Design review of the part shown in the three views and the two pictorial views. Dimensions are in mm from the part's minimum x, y and z. A direction names the side the tool comes from. Coordinates: 2 decimals unless noted, no trailing zeros. Order: outer loops, then holes, each group sorted by start corner. A loop starts at its lowest first (then second) coordinate and runs counter-clockwise, first axis right, second up. Notation, with made-up numbers: M -24,-32 L 16,-32 A31 cw 16,-6 Z; hole C -19.5,-29.5 d5. An arc over 180 degrees is marked long. Use CSV: the item, a comma, the result in double quotes.
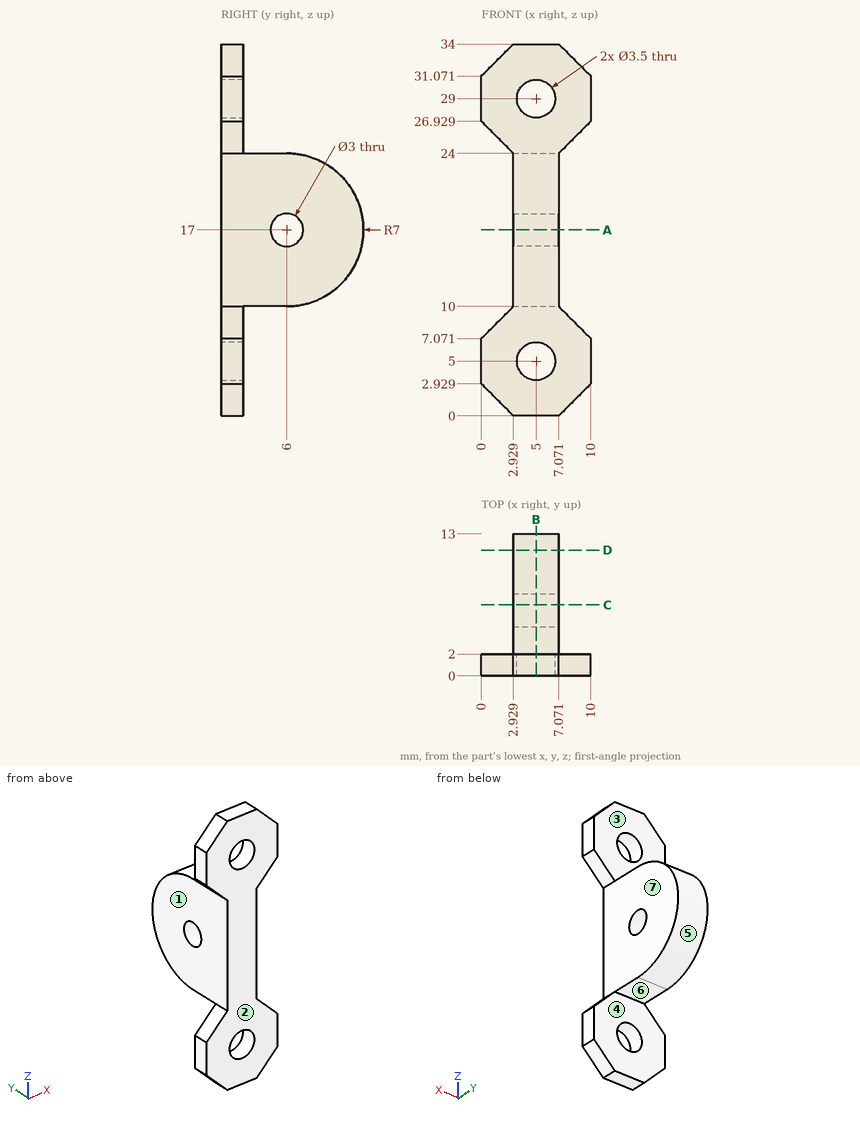
(1) The part is to be moulded in two halves that separate along Z. For the marked faces 4, 5, 6 and 7, say which applies: pulls with the +Z half, pulls with the -Z half, needs draft (parallel to the pull), parting line crosses it, or undercut.
The answers:
face 4,"needs draft"
face 5,"parting line crosses it"
face 6,"pulls with the -Z half"
face 7,"undercut"
(2) Wall thickness on probe 1 along X at (y, z) = (0.5, 29); probe 2 along X at (y, z) = (2, 11); probe 3 along Y at (x, z) = (3.8, 17): over which ranges is each line inside the solid? List them lowest first.
The answers:
probe 1,"x = 0 to 3.25, 6.75 to 10"
probe 2,"x = 2.93 to 7.07"
probe 3,"y = 0 to 4.5, 7.5 to 13"
(3) For the marked faces 1, 2 and 3, list the 3-axis set-ups (+Z, -Z, +X, -X, +Y, -Y) from which the entire face can be reached by the end or side of a thin tool; tool diameter is ignored.
The answers:
face 1,"-X, +Y, -Y"
face 2,"+Z, -Z, +X, -X, -Y"
face 3,"+Z, +X, -X, +Y"
(4) Add section C-C on y = 6.5. State the section outline as (x, z) points, and give its area (3 significant figures).
The answers:
outline,"M 2.93,10.02 L 7.07,10.02 L 7.07,15.59 L 2.93,15.59 Z; M 2.93,18.41 L 7.07,18.41 L 7.07,23.98 L 2.93,23.98 Z"
area,"46.1 mm2"
(5) Clearance check with flat-ended pins moving along their axes: P1, Ø6.5, axis at y = 6, z = 20, coming from the -X side; P2, Ø4.5, axis at x = 5, z = 29, coming from the +Y side; P3, Ø2.5, axis at y = 6, z = 17, coming from the +X side; P4, Ø3, axis at x = 5.5, y = 3, coming from the +Z side. State where each tip first meets the part, or that it passes through.
The answers:
P1,"stops at x = 2.93"
P2,"stops at y = 2"
P3,"passes through"
P4,"stops at z = 34"
(6) Add section B-B on x = 5. State the section outline as (y, z) points.
The answers:
outline,"M 0,0 L 2,0 L 2,3.25 L 0,3.25 Z; M 0,6.75 L 2,6.75 L 2,10 L 6,10 A7 ccw 6,24 L 2,24 L 2,27.25 L 0,27.25 Z; M 0,30.75 L 2,30.75 L 2,34 L 0,34 Z; hole C 6,17 d3"
(7) Add section A-A on z = 17. State the section outline as (x, y) points, and give its area (3 significant figures).
The answers:
outline,"M 2.93,0 L 7.07,0 L 7.07,4.5 L 2.93,4.5 Z; M 2.93,7.5 L 7.07,7.5 L 7.07,13 L 2.93,13 Z"
area,"41.4 mm2"
(8) Add section D-D on y = 11.5. State the section outline as (x, z) points.
The answers:
outline,"M 2.93,12.67 L 7.07,12.67 L 7.07,21.33 L 2.93,21.33 Z"
